```python
from build123d import *

# Parameters (mm, degrees)
EXTRUDE_THIN2_DEPTH = 279.4
FILLET1_R           = 1.651


with BuildPart() as part:
    # Sketch1 → Extrude-Thin2 (new body)
    with BuildSketch(Plane.XY):
        with BuildLine():
            Line((0, 0), (-0.6985, 0))
            ThreePointArc((-0.6985, 0), (-3.126908, 1.990818), (-1.651, 4.7625))
            Line((-1.651, 4.7625), (-1.651, 10.215706))
            ThreePointArc((-1.651, 10.215706), (-2.928564, 14.534173), (-6.35, 17.4625))
            Line((-6.35, 17.4625), (-6.35, 20.6375))
            ThreePointArc((-6.35, 20.6375), (-11.96266, 22.96234), (-14.2875, 28.575))
            Line((-14.2875, 28.575), (-17.4625, 28.575))
            Line((-17.4625, 28.575), (-17.4625, 41.275))
            Line((-17.4625, 41.275), (0, 41.275))
            Line((0, 41.275), (0, 39.624))
            Line((0, 39.624), (-15.8115, 39.624))
            Line((-15.8115, 39.624), (-15.8115, 30.226))
            Line((-15.8115, 30.226), (-12.415829, 30.226))
            ThreePointArc((-12.415829, 30.226), (-10.795227, 24.129773), (-4.699, 22.509171))
            Line((-4.699, 22.509171), (-4.699, 18.463865))
            ThreePointArc((-4.699, 18.463865), (-1.257164, 14.962092), (0, 10.215706))
            Line((0, 10.215706), (0, 2.916441))
            ThreePointArc((0, 2.916441), (-1.421211, 2.875423), (-0.6985, 1.651))
            Line((-0.6985, 1.651), (0, 1.651))
            Line((0, 1.651), (0, 0))
        make_face()
    extrude(amount=-EXTRUDE_THIN2_DEPTH)

    # Fillet1
    fillet1_edges = [part.edges().sort_by_distance(p)[0] for p in [
        (-12.415829, 30.226, -139.7),
        (-4.699, 22.509171, -139.7),
        (0, 2.916441, -139.7),
        (-6.35, 17.4625, -139.7),
        (-17.4625, 28.575, -139.7),
        (-17.4625, 41.275, -139.7),
    ]]
    fillet(fillet1_edges, radius=FILLET1_R)


solid = part.part
```
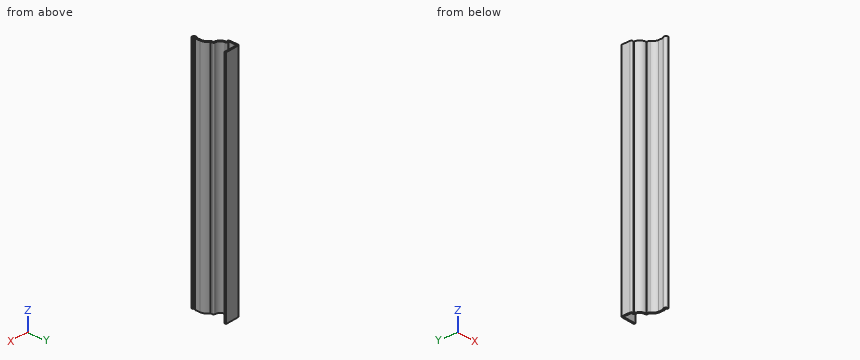
Design review of the part built by this model. Coordinates are the model's own, in mm. Give positions to 0.01 mm unless a question says otherwise; leave off trailing zeros. Loops run counter-clockwise (first coordinate to the right, second up) from the corner with the lowest first, then second, coordinate; pieces in that order, holes last. Notation, with made-up numbers: M -15.75,0.25 L 23.25,0.25 A31 ccw 23.25,25.25 Z; hole C 68.25,-16 d6. An arc over 180 degrees is marked long. Return JSON: item names as keys, results as strings. Group by question number.
Item 1: For probe 1 along Y at (x, z) = (-14.5, -187) (3 decimals); probe 2 along Y at (x, z) = (-13.5, -29.5) (3 decimals); probe 3 along X at (y, z) = (10, -84), list the stretches that pass through material, from the lowest coordinate up.
Item 2: Insertion check: pin 1 Ø1.6 at (y, z) = (8, -77.5) entering from -X; pin 2 Ø0.7 at (y, z) = (19.5, -184) entering from -X; pin 3 Ø8 at (y, z) = (6.5, -179.5) entering from -X; pin 4 Ø7.5 at (y, z) = (36, -150.5) entering from +X. Each pin has a flat end and moves straight along its axis. Give the tip position at first contact, or say it passes through.
Item 3: We need section B-B (y = 14). Give the boundary of the cut face in (x, z).
Output:
{
 "1": {"probe 1": "y = 28.575 to 30.226, 39.624 to 41.275", "probe 2": "y = 25.128 to 30.026, 39.624 to 41.275", "probe 3": "x = -1.65 to 0"},
 "2": {"pin 1": "stops at x = -1.65", "pin 2": "stops at x = -6.35", "pin 3": "stops at x = -3.17", "pin 4": "stops at x = 0"},
 "3": {"outline": "M -2.61,-279.4 L -0.78,-279.4 L -0.78,0 L -2.61,0 Z"}
}
